Geometry check sheet. Reference: the model listing, model coordinates, mm. A direction names the side the tool comes from. Give positions to 0.01 mm unless a question says otherwise; leave off trailing zeros. Loops run counter-clockwise (first coordinate to the right, second up) from the corner with the lowest first, then second, coordinate; pieces in that order, holes last. Notation, with made-up numbers: (20.5, 72) -> (36.5, 72) arc R3 cw to (36.5, 76) -> close; hole circle Ø2 at (73.5, 11). An arc over 180 degrees is marked (long way). One line per question, with ' | ' between items.
from build123d import *


with BuildPart() as part:
    # Sketch1 → Revolve1 (revolve)
    with BuildSketch(Plane.XY, mode=Mode.PRIVATE) as revolve1_sk:
        Polygon((-54, 0), (946, 0), (946, 5), (944.15, 5), (944.15, 4.8), (943, 4.8), (943, 5), (935, 5), (935, 8), (0, 8), (0, 6), (-25, 6), (-25, 5), (-27, 5), (-27, 6), (-39, 6), (-39, 5), (-54, 5), align=None)
    revolve(revolve1_sk.sketch.rotate(Axis((-54, 0, 0), (1, 0, 0)), 90), axis=Axis((-54, 0, 0), (1, 0, 0)))


solid = part.part
Item 1: Sectioned sample at C-C (x = 416). Record the cut outline in (y, z), plus the area to 3 significant figures.
Result:
outline: circle Ø16 at (0, 0) | area: 201 mm2
Item 2: Depth check by flat-ended pin: pin 1 Ø1 at (x, z) = (232, 2) entering from +Y; pin 2 Ø4 at (x, y) = (302, -4.5) entering from -Z; pin 3 Ø5 at (y, z) = (5.5, 5.5) entering from -X. Enter the tip coordinate at first touch or a pass-through.
Result:
pin 1: y = 7.86 | pin 2: z = -7.6 | pin 3: x = -39
Item 3: Set-up check for faces 1 (the face through (935, -0.1, -5.2)), 2 (the face through (460.96, 7.81, -1.73)), 3 (the face through (0, -6, -2)): record each of +Z, -Z, +X, -X, +Y, -Y from which the full face is reachable in a straight line by a thin tool's end or side.
Result:
face 1: +X | face 2: +X, -X | face 3: -X
Item 4: Scan lines: probe 1 along X at (y, z) = (3.75, -3.75); probe 2 along Y at (x, z) = (560.5, -1.5); probe 3 along Y at (x, z) = (565.5, -6.5). Record each from-to range of solid material in increasing order.
Result:
probe 1: -39 to -27, -25 to 935 | probe 2: -7.86 to 7.86 | probe 3: -4.66 to 4.66
